from build123d import *

# Parameters (mm, degrees)
F0_W      = 120
F0_H      = 130
F1_DEPTH  = 4
F3_DEPTH  = 10
F4_R      = 2
F5_DEPTH  = 5
F6_R      = 2
F7_DEPTH  = 135
F8_R      = 2
F9_DEPTH  = 5
F10_W     = 20
F10_H     = 10
F11_DEPTH = 5


with BuildPart() as f1:
    # F0 (on Top) → F1 (new body)
    with BuildSketch(Plane.XY):
        with Locations((-37.729894, -24.004591)):
            Rectangle(F0_W, F0_H)
    extrude(amount=F1_DEPTH)

    # F2 (on face) → F3 (join)
    with BuildSketch(Plane.XY.offset(4)):
        Polygon((-87.729894, -86.004591), (-87.729894, -89.004591), (22.270106, -89.004591), (22.270106, 40.995409), (-87.729894, 40.995409), (-87.729894, 37.995409), (19.270106, 37.995409), (19.270106, -86.004591), align=None)
    extrude(amount=F3_DEPTH)

    # F4 (on face) → F5 (cut)
    with BuildSketch(Plane.XY.offset(4)):
        with Locations((-92.729894, -21.004591)):
            Circle(F4_R)
        with Locations((-92.729894, -71.004591)):
            Circle(F4_R)
        with Locations((-92.729894, 22.995409)):
            Circle(F4_R)
    extrude(amount=-F5_DEPTH, mode=Mode.SUBTRACT)

    # F6 (on face) → F7 (cut)
    with BuildSketch(Plane.XZ.offset(89.004591)):
        with Locations((4.270106, 9)):
            Circle(F6_R)
        with Locations((-37.729894, 9)):
            Circle(F6_R)
        with Locations((-79.729894, 9)):
            Circle(F6_R)
    extrude(amount=-F7_DEPTH, mode=Mode.SUBTRACT)

    # F8 (on face) → F9 (cut)
    with BuildSketch(Plane.YZ.offset(22.270106)):
        with Locations((-71.004591, 9)):
            Circle(F8_R)
        with Locations((-24.004591, 9)):
            Circle(F8_R)
        with Locations((22.995409, 9)):
            Circle(F8_R)
    extrude(amount=-F9_DEPTH, mode=Mode.SUBTRACT)

    # F10 (on face) → F11 (cut)
    with BuildSketch(Plane.XY):
        with Locations((-52.729894, -34.004591)):
            Rectangle(F10_W, F10_H)
    extrude(amount=F11_DEPTH, mode=Mode.SUBTRACT)


solid = f1.part
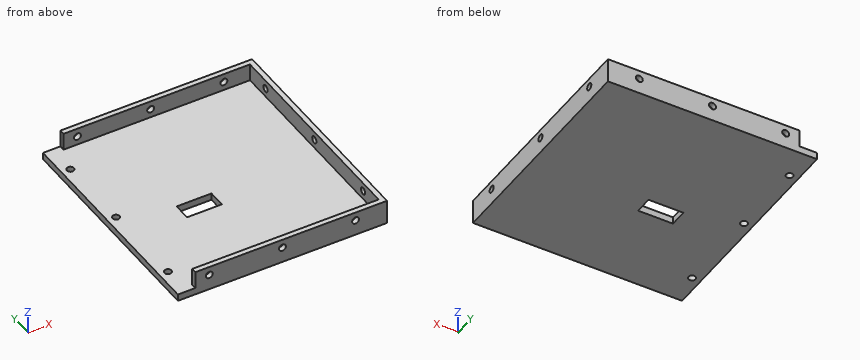
Design review of the part built by this model. Coordinates are the model's own, in mm. Give positions to 0.01 mm unless a question says otherwise; leave off trailing zeros. Order: outer loops, then holes, each group sorted by start corner. A loop starts at its lowest first (then second) coordinate and runs counter-clockwise, first axis right, second up. Notation, with made-up numbers: (75.5, 42) - (107.5, 42) arc R30 ccw to (107.5, 65) - close; hole circle Ø7 at (17.5, 72.5). An arc over 180 degrees is marked (long way). Write item = value, one per line. Start each with the question number.
Q1. Clearance check with flat-ended pins moving along their axes: pin 1 Ø4.5 at (x, z) = (-79.73, 9) entering from +Y; pin 2 Ø1.5 at (y, z) = (-88, 7.5) entering from -X; pin 3 Ø6 at (x, y) = (-39, -22) entering from +Z. State where each tip first meets the part, or that it passes through.
Q2. We need section A-A on x = -59.5. State the section outline as (y, z) points, plus the area to 3 significant figures.
Q3. We need section B-B on z = 2. State the section outline as (x, y) points.
Q4. To check wall thickness, follow L1, parallel to Y at x = -47, z = 6.5; L2, parallel to Z at x = 6, y = -71; L3, parallel to X at y = -22, z = 8. State the ranges of each line that lie inside material, in increasing order. Write a range as from..to.
Q5. We need section C-C on y = -6.5. State the section outline as (x, z) points.
Q6. We need section D-D on x = -22. State the section outline as (y, z) points.
Working result:
q1.pin_1 = 41
q1.pin_2 = -87.73
q1.pin_3 = 4
q2.outline = (-89, 0) - (-39, 0) - (-39, 4) - (-86, 4) - (-86, 14) - (-89, 14) - close; (-29, 0) - (41, 0) - (41, 14) - (38, 14) - (38, 4) - (-29, 4) - close
q2.area = 540 mm²
q3.outline = (-97.73, -89) - (22.27, -89) - (22.27, 41) - (-97.73, 41) - close; hole circle Ø4 at (-92.73, -71); hole circle Ø4 at (-92.73, -21); hole circle Ø4 at (-92.73, 23); hole (-62.73, -39) - (-42.73, -39) - (-42.73, -29) - (-62.73, -29) - close
q4.L1 = -89..-86, 38..41
q4.L2 = 0..4
q4.L3 = 19.27..22.27
q5.outline = (-97.73, 0) - (22.27, 0) - (22.27, 14) - (19.27, 14) - (19.27, 4) - (-97.73, 4) - close
q6.outline = (-89, 0) - (41, 0) - (41, 14) - (38, 14) - (38, 4) - (-86, 4) - (-86, 14) - (-89, 14) - close
